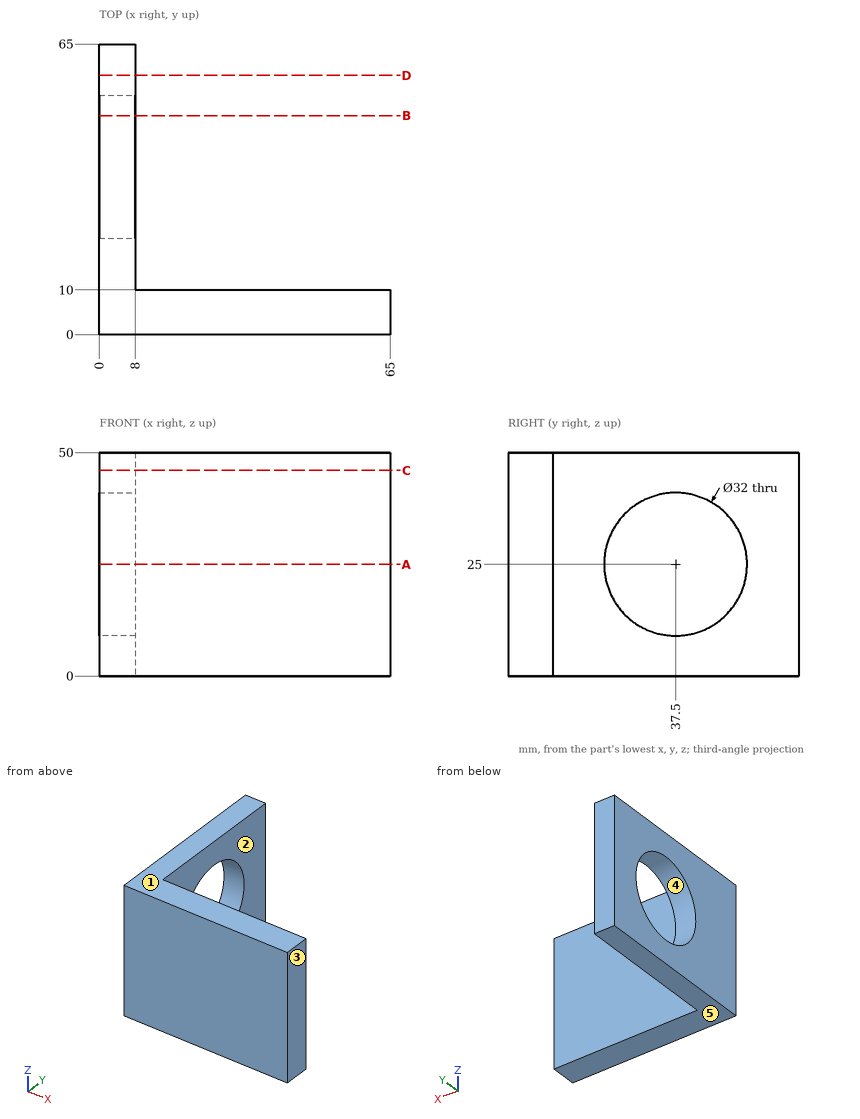
Source: three-view drawing plus pictorial views. Frame: mm from the lowest corner of the part. A direction names the side the tool comes from. Round coordinates to 2 decimals unless told otherwise and drop trailing zeros. Loops run counter-clockwise (first coordinate to the right, second up) from the corner with the lowest first, then second, coordinate; pieces in that order, holes last. Notation, with made-up numbers: M 43.5,18 L 66.5,18 A31 ccw 66.5,45 Z; hole C 21.5,78 d4. An arc over 180 degrees is marked long. Put each result on its own line as item: value.
(1) Access query for the marked faces 1 and 2. Directions: +Z, -Z, +X, -X, +Y, -Y. A direction counts if a zero-diameter tool reaches every point of the face in a straight line with its end or side. Return the directions, or none.
Solutions:
face 1: +Z, +X, -X, +Y, -Y
face 2: +Z, -Z, +X, +Y
(2) Pull-direction query (Z, two-part tool) for the marked faces 3, 4 and 5; classes: released by +Z, released by -Z, zero draft, split by the parting line, or undercut.
Solutions:
face 3: zero draft
face 4: undercut
face 5: released by -Z
(3) First-contact query: pin 1 (25 mm diameter, centred on y = 34, z = 24.5, fed in from +X); pin 2 (4 mm diameter, centred on x = 47.5, y = 11.5, fed in from -Z); pin 3 (8 mm diameter, centred on x = 20.5, z = 31.5, fed in from +Y). Flat tips, straight axial feed; report the tip coordinate or a pass-through.
Solutions:
pin 1: x = 8
pin 2: z = 0
pin 3: y = 10
(4) Section B-B, the plane y = 49. Return loops of the section in (x, z), and give its area (3 significant figures).
Solutions:
outline: M 0,0 L 8,0 L 8,13.88 L 0,13.88 Z; M 0,36.12 L 8,36.12 L 8,50 L 0,50 Z
area: 222 mm²
(5) Section D-D, the plane y = 58. Return loops of the section in (x, z), and give its area (3 significant figures).
Solutions:
outline: M 0,0 L 8,0 L 8,50 L 0,50 Z
area: 400 mm²
(6) Section C-C, the plane z = 46. Return loops of the section in (x, y).
Solutions:
outline: M 0,0 L 65,0 L 65,10 L 8,10 L 8,65 L 0,65 Z
(7) Section A-A, the plane z = 25. Return loops of the section in (x, y), and give its area (3 significant figures).
Solutions:
outline: M 0,0 L 65,0 L 65,10 L 8,10 L 8,21.5 L 0,21.5 Z; M 0,53.5 L 8,53.5 L 8,65 L 0,65 Z
area: 834 mm²
(8) Ray query, line 1 (Z direction, x = 6, y = 37); line 2 (X direction, y = 48.5, z = 6); line 3 (Y direction, x = 33, z = 40). Return the intervals inside material, ascending. Write a range as [from, to].
Solutions:
line 1: [0, 9.01], [40.99, 50]
line 2: [0, 8]
line 3: [0, 10]
